Model file for the job. Use its own axes, mm. Coordinates: 2 decimals unless noted, no trailing zeros. Order: outer loops, then holes, each group sorted by start corner. A loop starts at its lowest first (then second) coordinate and runs counter-clockwise, first axis right, second up. Notation, with made-up numbers: M 56,40.25 L 113,40.25 A14 cw 113,58.25 Z; hole C 51,66 d3. An arc over 180 degrees is marked long. Return JSON: item names as keys, results as strings.
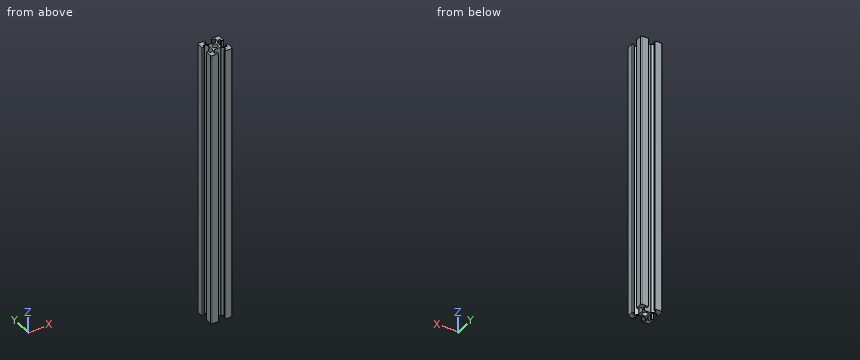
```python
from build123d import *

# Parameters (mm, degrees)
SKETCH1_R           = 2.5
BOSS_EXTRUDE1_DEPTH = 300
FILLET1_R           = 1
FILLET2_R           = 0.5
FILLET3_R           = 0.5
FILLET4_R           = 0.5
FILLET5_R           = 0.5
SKETCH4_W           = 85.130466005
SKETCH4_H           = 76.492403511
CUT_EXTRUDE4_DEPTH  = 40


with BuildPart() as part:
    # Sketch1 → Boss-Extrude1 (new body)
    with BuildSketch(Plane.XY):
        Polygon((13.2, 0), (13.2, 1.8), (15.45, 1.8), (15.45, 3.6), (12.95, 6.1), (7.05, 6.1), (4.55, 3.6), (4.55, 1.8), (6.8, 1.8), (6.8, 0), (0, 0), (0, 6.8), (1.8, 6.8), (1.8, 4.55), (3.6, 4.55), (6.1, 7.05), (6.1, 12.95), (3.6, 15.45), (1.8, 15.45), (1.8, 13.2), (0, 13.2), (0, 20), (6.8, 20), (6.8, 18.2), (4.55, 18.2), (4.55, 16.4), (7.05, 13.9), (12.95, 13.9), (15.45, 16.4), (15.45, 18.2), (13.2, 18.2), (13.2, 20), (20, 20), (20, 13.2), (18.2, 13.2), (18.2, 15.45), (16.4, 15.45), (13.9, 12.95), (13.9, 7.05), (16.4, 4.55), (18.2, 4.55), (18.2, 6.8), (20, 6.8), (20, 0), align=None)
        with Locations((10, 10)):
            Circle(SKETCH1_R, mode=Mode.SUBTRACT)
    extrude(amount=BOSS_EXTRUDE1_DEPTH)

    # Fillet1
    fillet1_edges = [part.edges().sort_by_distance(p)[0] for p in [
        (0, 0, 150),
        (0, 20, 150),
        (20, 20, 150),
        (20, 0, 150),
    ]]
    fillet(fillet1_edges, radius=FILLET1_R)

    # Fillet2
    fillet2_edges = [part.edges().sort_by_distance(p)[0] for p in [
        (4.55, 18.2, 150),
        (4.55, 16.4, 150),
        (7.05, 13.9, 150),
        (12.95, 13.9, 150),
        (15.45, 16.4, 150),
        (15.45, 18.2, 150),
    ]]
    fillet(fillet2_edges, radius=FILLET2_R)

    # Fillet3
    fillet3_edges = [part.edges().sort_by_distance(p)[0] for p in [
        (18.2, 15.45, 150),
        (16.4, 15.45, 150),
        (13.9, 12.95, 150),
        (13.9, 7.05, 150),
        (16.4, 4.55, 150),
        (18.2, 4.55, 150),
    ]]
    fillet(fillet3_edges, radius=FILLET3_R)

    # Fillet4
    fillet4_edges = [part.edges().sort_by_distance(p)[0] for p in [
        (1.8, 4.55, 150),
        (3.6, 4.55, 150),
        (6.1, 7.05, 150),
        (6.1, 12.95, 150),
        (3.6, 15.45, 150),
        (1.8, 15.45, 150),
    ]]
    fillet(fillet4_edges, radius=FILLET4_R)

    # Fillet5
    fillet5_edges = [part.edges().sort_by_distance(p)[0] for p in [
        (15.45, 1.8, 150),
        (15.45, 3.6, 150),
        (12.95, 6.1, 150),
        (7.05, 6.1, 150),
        (4.55, 3.6, 150),
        (4.55, 1.8, 150),
    ]]
    fillet(fillet5_edges, radius=FILLET5_R)

    # Sketch4 → Cut-Extrude4 (cut)
    with BuildSketch(Plane(origin=(0, 0, 0), x_dir=(-1, 0, 0), z_dir=(0, 0, -1))):
        with Locations((13.179490335, -10.50880322)):
            Rectangle(SKETCH4_W, SKETCH4_H)
    extrude(amount=-CUT_EXTRUDE4_DEPTH, mode=Mode.SUBTRACT)


solid = part.part
```
Item 1: Wall check: line 1 (Y direction, x = 18, z = 54.5); line 2 (X direction, y = 14, z = 103); line 3 (X direction, y = 17.5, z = 174.5). Give the ranges that are in metal, low to high.
Check result:
{"line 1": "y = 0 to 4.65, 15.35 to 20", "line 2": "x = 0 to 1.8, 5.05 to 6.96, 13.04 to 14.95, 18.2 to 20", "line 3": "x = 0 to 4.55, 15.45 to 20"}
Item 2: Drop flat-ended pins along their axis: pin 1 Ø1.6 at (y, z) = (11.5, 107) entering from +X; pin 2 Ø1.6 at (x, z) = (10.5, 198.5) entering from +Y; pin 3 Ø2 at (x, z) = (11.5, 76.5) entering from -Y. Give the stop position or say it passes through.
Check result:
{"pin 1": "stops at x = 13.9", "pin 2": "stops at y = 13.9", "pin 3": "stops at y = 6.1"}
Item 3: Saw through at A-A (x = 10). Write the cut outline in (y, z), and give its area (3 significant figures).
Check result:
{"outline": "M 6.1,40 L 7.5,40 L 7.5,300 L 6.1,300 Z; M 12.5,40 L 13.9,40 L 13.9,300 L 12.5,300 Z", "area": "728 mm2"}
